Geometry: final body of the model. Coordinates: model frame, mm. Face numbers are marked on the shaded views. Give positions to 0.01 mm unless a question says otherwise; leave off trailing zeros. Write each loop counter-clockwise with the first axis right and the second up, starting at its lowest first coordinate (ties: lowest second). Pieces come first, ordered by that corner, then holes. Notation, with made-up numbers: M 84.5,32.5 L 113.5,32.5 A18 ccw 113.5,63.5 Z; hole C 22,51.25 d1. An arc over 180 degrees is marked long. Answer as a JSON object with one key per item and string values.
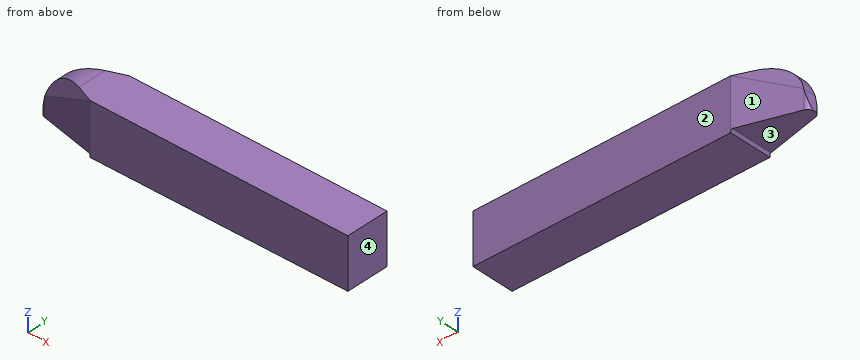
from build123d import *

# Parameters (mm, degrees)
EXTRUDE_1_DEPTH     = 24
SKETCH_2_OUTSIDE_W  = 182.644
SKETCH_2_OUTSIDE_H  = 56.644
CUT_EXTRUDE_1_DEPTH = 24
SKETCH_6_W          = 43.637196822
SKETCH_6_H          = 35.300538325
CUT_EXTRUDE_2_DEPTH = 24


with BuildPart() as part:
    # Эскиз1 → Бобышка-Вытянуть1 (new body)
    with BuildSketch(Plane.XY):
        with BuildLine():
            Line((0, 0), (120, 0))
            Line((120, 0), (120, 20))
            Line((120, 20), (0, 20))
            Line((0, 20), (-27.743147483, 12.906498205))
            ThreePointArc((-27.743147483, 12.906498205), (-30, 10), (-27.743147483, 7.093501795))
            Line((-27.743147483, 7.093501795), (0, 0))
        make_face()
    extrude(amount=EXTRUDE_1_DEPTH)

    # Эскиз2 outside → Вырез-Вытянуть1 (cut)
    with BuildSketch(Plane(origin=(0, 0, 0), x_dir=(1, 0, 0), z_dir=(0, 1, 0))):
        with Locations((45, -12)):
            Rectangle(SKETCH_2_OUTSIDE_W, SKETCH_2_OUTSIDE_H)
        with BuildLine():
            Line((-30, 0), (-27.541196148, -9.176380902))
            ThreePointArc((-27.541196148, -9.176380902), (-20.397908202, -19.867066806), (-8.222679622, -24))
            Line((-8.222679622, -24), (0, -24))
            Line((0, -24), (155.035600822, -24))
            Line((155.035600822, -24), (155.035600822, -0.765531499))
            Line((155.035600822, -0.765531499), (0, 0))
            Line((0, 0), (0, -0.765531499))
            ThreePointArc((0, -0.765531499), (-0.238574389, -1.320828429), (-0.805596322, -1.530013864))
            Line((-0.805596322, -1.530013864), (-30, 0))
        make_face(mode=Mode.SUBTRACT)
    extrude(amount=CUT_EXTRUDE_1_DEPTH, mode=Mode.SUBTRACT)

    # Эскиз6 → Вырез-Вытянуть2 (cut)
    with BuildSketch(Plane(origin=(-8.581317892, 21.458428849, 5.749768681), x_dir=(0.9328250222338894, 0.34805174336163447, 0.09326018355799502), z_dir=(-0.36032967945250355, 0.9010397803843876, 0.24143288150231465))):
        with Locations((-5.019191461, -7.289608273)):
            Rectangle(SKETCH_6_W, SKETCH_6_H)
    cut_extrude_2 = extrude(amount=CUT_EXTRUDE_2_DEPTH, mode=Mode.SUBTRACT)

    # Зеркальное отражение1: Вырез-Вытянуть2 across plane
    add(cut_extrude_2.mirror(Plane(origin=(0, 10, 0), x_dir=(0, 0, 1), z_dir=(0, -1, 0))), mode=Mode.SUBTRACT)


solid = part.part
1) Cut plane A-A on z = 22.25. Return loops of the section in (x, y).
Geometry check:
{"outline": "M -16.4,6.09 L -3.25,0.83 L 0,0 L 120,0 L 120,20 L 0,20 L -3.25,19.17 L -16.4,13.91 Z"}
2) Pull-direction query (X, two-part tool) for the marked faces 1, 2, 3 and 4; classes: pulls with the +X half, pulls with the -X half, needs draft (parallel to the pull), parting line crosses it, or undercut.
Geometry check:
{"face 1": "pulls with the -X half", "face 2": "needs draft", "face 3": "undercut", "face 4": "pulls with the +X half"}
3) Cut plane D-D on x = 89. Return loops of the section in (y, z).
Geometry check:
{"outline": "M 0,0.44 L 20,0.44 L 20,24 L 0,24 Z"}
4) Line query: line 1 (Z direction, x = 2, y = 3.25); line 2 (Z direction, x = 114, y = 15.5); line 3 (X direction, y = 8.5, z = 20.25). Output: solid intervals per line, ascending. Write a range as from..to.
Geometry check:
{"line 1": "z = 0.01..24", "line 2": "z = 0.56..24", "line 3": "x = -19.88..120"}
5) Contact query for flat-ended pins moving along their axis: P1, Ø8, axis at x = 7, y = 10, coming from the -Z side; P2, Ø1, axis at x = 45, y = 11, coming from the -Z side; P3, Ø1.5, axis at x = -10.5, y = 14.5, coming from the +Z side. Output: stop coordinate, or through.
Geometry check:
{"P1": "stops at z = 0.01", "P2": "stops at z = 0.22", "P3": "stops at z = 23.94"}
6) Cut plane C-C on z = 13.75. Return loops of the section in (x, y), and give its area (3 significant figures).
Geometry check:
{"outline": "M -25.69,7.53 L -19.04,4.87 L 0,0 L 120,0 L 120,20 L 0,20 L -19.04,15.13 L -25.69,12.47 Z", "area": "2,740 mm2"}
7) Cut plane B-B on x = -3. Return loops of the section in (y, z), and give its area (3 significant figures).
Geometry check:
{"outline": "M 0.77,1.42 L 19.23,1.42 L 19.23,22.39 L 18.8,24 L 1.2,24 L 0.77,22.39 Z", "area": "416 mm2"}
